Geometry: final body of the model. Coordinates: model frame, mm. Coordinates: 2 decimals unless noted, no trailing zeros. Write each loop counter-clockwise with the first axis right and the second up, starting at its lowest first coordinate (ties: lowest second). Pieces come first, ordered by that corner, then holes. Notation, with made-up numbers: (75, -26) -> (111, -26) arc R28 cw to (111, 1) -> close; hole circle Ø8 at (-29.75, 35.5). An arc over 180 degrees is marked (long way). One line per item, written item: value.
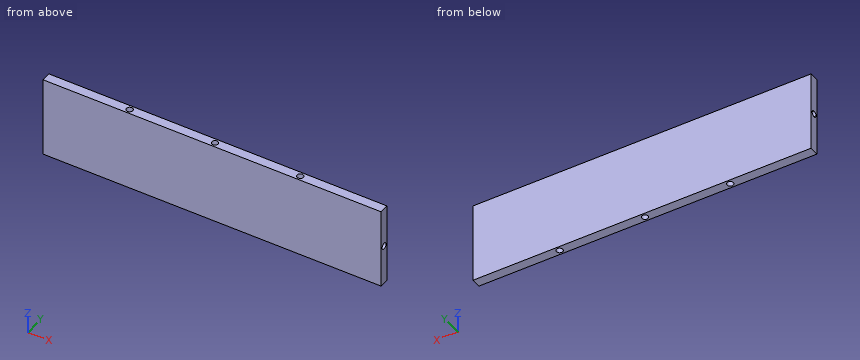
```python
from build123d import *

# Parameters (mm, degrees)
F0_W     = 216.049
F0_H     = 51.69
F1_DEPTH = 6
F2_R     = 2
F3_DEPTH = 10
F5_DEPTH = 10
F6_START = -45.69
F6_DEPTH = 6
F7_DEPTH = 10
F8_R     = 2
F9_DEPTH = 10


with BuildPart() as f1:
    # F0 (on Front) → F1 (new body)
    with BuildSketch(Plane.XZ):
        with Locations((0, 25.845)):
            Rectangle(F0_W, F0_H)
    extrude(amount=F1_DEPTH)

    # F2 (on face) → F3 (cut)
    with BuildSketch(Plane(origin=(0, 0, 0), x_dir=(1, 0, 0), z_dir=(0, 0, -1))):
        with Locations((0, 3)):
            Circle(F2_R)
        with Locations((-54.5, 3)):
            Circle(F2_R)
        with Locations((54.5, 3)):
            Circle(F2_R)
    extrude(amount=-F3_DEPTH, mode=Mode.SUBTRACT)

    # F4 (on face) → F5 (join)
    with BuildSketch(Plane(origin=(-108.0245, 0, 0), x_dir=(0, -1, 0), z_dir=(-1, 0, 0))):
        with BuildLine():
            ThreePointArc((5, 25.845), (4.4142135624, 27.2592135624), (3, 27.845))
            Line((3, 27.845), (3, 23.845))
            ThreePointArc((3, 23.845), (4.4142135624, 24.4307864376), (5, 25.845))
        make_face()
        with BuildLine():
            Line((3, 23.845), (3, 27.845))
            ThreePointArc((3, 27.845), (1, 25.845), (3, 23.845))
        make_face()
    extrude(amount=-F5_DEPTH)

    # F2 (on face) → F6 (cut)
    with BuildSketch(Plane(origin=(0, 0, 0), x_dir=(1, 0, 0), z_dir=(0, 0, -1)).offset(F6_START)):
        with Locations((0, 3)):
            Circle(F2_R)
        with Locations((-54.5, 3)):
            Circle(F2_R)
        with Locations((54.5, 3)):
            Circle(F2_R)
    extrude(amount=-F6_DEPTH, mode=Mode.SUBTRACT)

    # F4 (on face) → F7 (cut)
    with BuildSketch(Plane(origin=(-108.0245, 0, 0), x_dir=(0, -1, 0), z_dir=(-1, 0, 0))):
        with BuildLine():
            Line((3, 23.845), (3, 27.845))
            ThreePointArc((3, 27.845), (1, 25.845), (3, 23.845))
        make_face()
        with BuildLine():
            ThreePointArc((5, 25.845), (4.4142135624, 27.2592135624), (3, 27.845))
            Line((3, 27.845), (3, 23.845))
            ThreePointArc((3, 23.845), (4.4142135624, 24.4307864376), (5, 25.845))
        make_face()
    extrude(amount=-F7_DEPTH, mode=Mode.SUBTRACT)

    # F8 (on face) → F9 (cut)
    with BuildSketch(Plane.YZ.offset(108.0245)):
        with Locations((-3, 25.845)):
            Circle(F8_R)
    extrude(amount=-F9_DEPTH, mode=Mode.SUBTRACT)


solid = f1.part
```
(1) Line query: line 1 (X direction, y = -3, z = 8.25); line 2 (Y direction, x = -54.5, z = 48.5); line 3 (X direction, y = -1.2, z = 6). Output: solid intervals per line, ascending. Write a range as [from, to].
Responses:
line 1: x = [-108.02, -56.5], [-52.5, -2], [2, 52.5], [56.5, 108.02]
line 2: y = [-6, -5], [-1, 0]
line 3: x = [-108.02, -55.37], [-53.63, -0.87], [0.87, 53.63], [55.37, 108.02]
(2) First-contact query: pin 1 (1.2 mm diameter, centred on y = -2.5, z = 26, fed in from -X); pin 2 (2 mm diameter, centred on x = 54.5, y = -2.5, fed in from -Z); pin 3 (1.2 mm diameter, centred on x = -54, y = -2.5, fed in from +Z); pin 4 (3 mm diameter, centred on y = -3, z = 26.5, fed in from +X). Flat tips, straight axial feed; report the tip coordinate or a pass-through.
Responses:
pin 1: stops at x = -98.02
pin 2: stops at z = 10
pin 3: stops at z = 45.69
pin 4: stops at x = 108.02
(3) Section A-A (z = 4.5). Return the cut outline in (x, y).
Responses:
outline: (-108.02, -6) -> (108.02, -6) -> (108.02, 0) -> (-108.02, 0) -> close; hole circle Ø4 at (-54.5, -3); hole circle Ø4 at (0, -3); hole circle Ø4 at (54.5, -3)
(4) Section B-B (x = -54.5). Return the cut outline in (y, z).
Responses:
outline: (-6, 0) -> (-5, 0) -> (-5, 10) -> (-1, 10) -> (-1, 0) -> (0, 0) -> (0, 51.69) -> (-1, 51.69) -> (-1, 45.69) -> (-5, 45.69) -> (-5, 51.69) -> (-6, 51.69) -> close
